Verification items for the finished model (mm, model axes). Face numbers are marked on the shaded views. A direction names the side the tool comes from. Round coordinates to 2 decimals unless told otherwise and drop trailing zeros. Order: outer loops, then holes, each group sorted by start corner. A loop starts at its lowest first (then second) coordinate and runs counter-clockwise, first axis right, second up. Notation, with made-up numbers: M 11.25,44 L 21.25,44 A34 cw 21.25,74 Z; hole C 57.5,28.25 d11. An arc over 180 degrees is marked long. One line per item, written item: value. Start each with the question number.
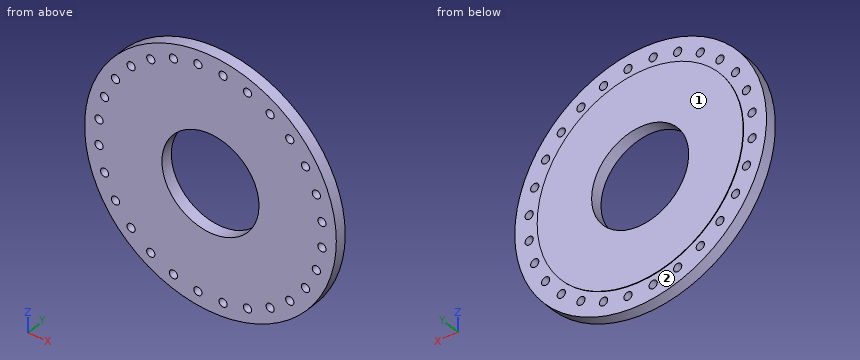
Solid Edge part; units mm, degrees
sketch "Sketch1" plane through (0, 0, 0) normal (0, -1, 0) x (1, 0, 0)
  circle A0 centre (0, 0) radius 376.5
  circle A1 centre (0, 0) radius 177.5
extrude "Protrusion1" add sketch "Sketch1" against normal blind 44.2
sketch "Sketch2" plane through (0, 0, 0) normal (0, -1, 0) x (1, 0, 0)
  circle A0 centre (0, 0) radius 460
  circle A1 centre (0, 0) radius 376.5
extrude "ProtrusiónExtruida_2" add sketch "Sketch2" against normal blind 42
hole "AGUJERO_30MM" at (-45.9054, 0, 407.422) direction (0, 1, 0) diameter 30 end up to next
pattern_circular "Pattern1" count 28 over 360 about axis through (0, 0, 0) along (0, 1, 0) of "AGUJERO_30MM"
1. Section check A-A (z = 0). Record the cut outline in (x, y), and give its area (3 significant figures).
2. Section check B-B (x = 0). Record the cut outline in (y, z).
3. Tool access check on the marked faces 1 and 2. Record the directions out of +Z, -Z, +X, -X, +Y, -Y that give a thin tool (end or side, any length) a straight path to the whole face; none if there is none.
4. Scan lines: line 1 along Z through (x, y) = (-37, 2.5); line 2 along X through (y, z) = (14, 126.5); line 3 along X through (y, z) = (9.5, -38). Record each from-to range of solid material in increasing order.
5. Depth check by flat-ended pin: pin 1 (1 mm diameter, centred on x = 308, y = 11.5, fed in from +Z); pin 2 (5 mm diameter, centred on x = -163.5, y = 19.5, fed in from +Z); pin 3 (12 mm diameter, centred on y = 24.5, z = -92, fed in from -X). Enter the tip coordinate at first touch or a pass-through.
Geometry check:
1. outline: M -460,0 L -177.5,0 L -177.5,44.2 L -376.5,44.2 L -376.5,42 L -460,42 Z; M 177.5,0 L 460,0 L 460,42 L 376.5,42 L 376.5,44.2 L 177.5,44.2 Z
1. area: 24,600 mm²
2. outline: M 0,-460 L 42,-460 L 42,-376.5 L 44.2,-376.5 L 44.2,-177.5 L 0,-177.5 Z; M 0,177.5 L 44.2,177.5 L 44.2,376.5 L 42,376.5 L 42,460 L 0,460 Z
3. face 1: +Z, -Z, +X, -X, +Y
3. face 2: +Y
4. line 1: z = -458.51 to -419.49, -395.35 to -173.6, 173.6 to 395.35, 419.49 to 458.51
4. line 2: x = -442.26 to -399.06, -374.93 to -124.52, 124.52 to 374.93, 399.06 to 442.26
4. line 3: x = -458.43 to -420.17, -394.67 to -173.38, 173.38 to 394.67, 420.17 to 458.43
5. pin 1: stops at z = 342.12
5. pin 2: stops at z = 430.9
5. pin 3: stops at x = -451.89
